from build123d import *

# Parameters (mm, degrees)
BOSS_EXTRUDE1_DEPTH = 20
SKETCH2_R           = 15.01
BOSS_EXTRUDE2_DEPTH = 20
CHAMFER1_SIZE       = 1
CHAMFER3_SIZE       = 1
SKETCH5_R           = 2.65
CUT_EXTRUDE2_DEPTH  = 40
FILLET3_R           = 5
SKETCH6_R           = 3.65
CUT_EXTRUDE3_DEPTH  = 8
CHAMFER4_SIZE       = 0.5
SKETCH10_R          = 15.01
BOSS_EXTRUDE5_DEPTH = 20
CHAMFER5_SIZE       = 1
SKETCH11_R          = 2.0099999999999967
CUT_EXTRUDE5_DEPTH  = 40
SKETCH12_R          = 2.0000000000000018
SKETCH12_R_2        = 2.000000000000005
SKETCH12_R_3        = 1.9999999999999967
CUT_EXTRUDE6_DEPTH  = 19.999999999999996


with BuildPart() as part:
    # Sketch1 → Boss-Extrude1 (new body)
    with BuildSketch(Plane(origin=(0, 0, 0), x_dir=(1, 0, 0), z_dir=(0, 1, 0))):
        with BuildLine():
            ThreePointArc((-23, 0), (1.41e-15, -22.999999999999982), (23, 0))
            ThreePointArc((23, 0), (17.845208734768505, 58.18386045047181), (20.033890701411753, 116.55459936267802))
            ThreePointArc((20.033890701411753, 116.55459936267802), (21.27316153822275, 124.05347023326534), (23.45051159720983, 131.33550314045155))
            ThreePointArc((23.45051159720983, 131.33550314045155), (-2.067e-14, 165.00000000000006), (-23.45051159720983, 131.3355031404515))
            ThreePointArc((-23.45051159720983, 131.3355031404515), (-21.27316153822273, 124.05347023326526), (-20.033890701411725, 116.55459936267786))
            ThreePointArc((-20.033890701411725, 116.55459936267786), (-17.845208734768505, 58.1838604504716), (-23, 0))
        make_face()
    extrude(amount=BOSS_EXTRUDE1_DEPTH)

    # Sketch2 → Boss-Extrude2 (add)
    with BuildSketch(Plane(origin=(0, 20, 0), x_dir=(1, 0, 0), z_dir=(0, 1, 0))):
        with Locations(Location((0, 0, 0), (0, 0, 90))):
            Circle(SKETCH2_R)
    extrude(amount=BOSS_EXTRUDE2_DEPTH)

    # Chamfer1
    chamfer1_edges = [part.edges().sort_by_distance(p)[0] for p in [
        (-2.76e-15, 40, 15.01),
    ]]
    chamfer(chamfer1_edges, length=CHAMFER1_SIZE)

    # Chamfer3
    # the kernel refuses this chamfer: 1 mm, written as the material it adds along each edge
    with BuildSketch(Plane(origin=(0, 20, 0), x_dir=(6e-17, 0, -1), z_dir=(1, 0, 6e-17))) as chamfer3_piece_1:
        Polygon((15.01, CHAMFER3_SIZE), (15.01 + CHAMFER3_SIZE, 0), (15.01, 0), align=None)
    revolve(axis=Axis((0, 20, 0), (0, 1, 0)))
    # the kernel refuses this chamfer: 1 mm, written as the material it takes off along each edge
    with BuildSketch(Plane(origin=(-79.73173943051358, 20, -110.54071067753486), x_dir=(0.9380204638883933, 0, -0.3465798743819428), z_dir=(-0.3465798743819428, 0, -0.9380204638883933))) as chamfer3_2_piece_1:
        Polygon((60.00000000000017 + CHAMFER3_SIZE, 0), (60.00000000000017, CHAMFER3_SIZE), (60.00000000000017, 0), align=None)
    revolve(axis=Axis((-79.73173943051358, 20, -110.54071067753486), (0, -1, 0)), revolution_arc=14.525766875036835, mode=Mode.SUBTRACT)
    with BuildSketch(Plane(origin=(-482.16572850262514, 20, -70.00000000000004), x_dir=(0.9949641454850282, 0, -0.1002314780857173), z_dir=(-0.1002314780857173, 0, -0.9949641454850282))) as chamfer3_2_piece_2:
        Polygon((464.4708454051196 + CHAMFER3_SIZE, 0), (464.4708454051196, CHAMFER3_SIZE), (464.4708454051196, 0), align=None)
    revolve(axis=Axis((-482.16572850262514, 20, -70.00000000000004), (0, -1, 0)), revolution_arc=14.737763084908373, mode=Mode.SUBTRACT)
    with BuildSketch(Plane(origin=(0, 20, -1.599e-14), x_dir=(-0.9937354343699007, 0, -0.11175816067592001), z_dir=(0.11175816067592001, 0, -0.9937354343699007))) as chamfer3_2_piece_3:
        Polygon((23.000000000000004 - CHAMFER3_SIZE, 0), (23.000000000000004, -CHAMFER3_SIZE), (23.000000000000004, 0), align=None)
    revolve(axis=Axis((0, 20, -1.599e-14), (0, 1, 0)), revolution_arc=192.83335153216495, mode=Mode.SUBTRACT)
    with BuildSketch(Plane(origin=(482.16572850261997, 20, -69.99999999999986), x_dir=(-0.9877285445231084, 0, 0.15618041597544133), z_dir=(0.15618041597544133, 0, 0.9877285445231084))) as chamfer3_2_piece_4:
        Polygon((464.4708454051149 + CHAMFER3_SIZE, 0), (464.47084540511446, CHAMFER3_SIZE), (464.4708454051149, 0), align=None)
    revolve(axis=Axis((482.16572850261997, 20, -69.99999999999986), (0, -1, 0)), revolution_arc=14.737763084908554, mode=Mode.SUBTRACT)
    with BuildSketch(Plane(origin=(79.7317394305139, 20, -110.54071067753493), x_dir=(-0.9949641454850281, 0, -0.10023147808571735), z_dir=(-0.10023147808571735, 0, 0.9949641454850281))) as chamfer3_2_piece_5:
        Polygon((60.000000000000455 + CHAMFER3_SIZE, 0), (60.000000000000455, CHAMFER3_SIZE), (60.000000000000455, 0), align=None)
    revolve(axis=Axis((79.7317394305139, 20, -110.54071067753493), (0, -1, 0)), revolution_arc=14.525766875036666, mode=Mode.SUBTRACT)
    with BuildSketch(Plane(origin=(9.77e-15, 20, -140.00000000000006), x_dir=(0.9380204638883942, 0, 0.3465798743819405), z_dir=(-0.3465798743819405, 0, 0.9380204638883942))) as chamfer3_2_piece_6:
        Polygon((24.999999999999982 - CHAMFER3_SIZE, 0), (24.999999999999982, -CHAMFER3_SIZE), (24.999999999999982, 0), align=None)
    revolve(axis=Axis((9.77e-15, 20, -140.00000000000006), (0, 1, 0)), revolution_arc=220.55653408148345, mode=Mode.SUBTRACT)

    # Sketch5 → Cut-Extrude2 (cut)
    with BuildSketch(Plane(origin=(0, 40, 0), x_dir=(1, 0, 0), z_dir=(0, 1, 0))):
        with Locations(Location((0, 0, 0), (0, 0, 270))):
            Circle(SKETCH5_R)
    extrude(amount=-CUT_EXTRUDE2_DEPTH, mode=Mode.SUBTRACT)

    # Fillet3
    # the kernel refuses this fillet: 5 mm, written as the material it takes off along each edge
    with BuildSketch(Plane(origin=(482.16572850261997, 0, -69.99999999999986), x_dir=(-0.9868985080370148, 0, 0.1613422909045059), z_dir=(0.1613422909045059, 0, 0.9868985080370148))) as fillet3_piece_1:
        with BuildLine():
            CenterArc((464.4708454051144 + FILLET3_R, -FILLET3_R), FILLET3_R, 89.99999999999935, 90.00000000000068)
            Line((464.4708454051144 + FILLET3_R, 8.9e-16), (464.4708454051144 + FILLET3_R, FILLET3_R * 0.02))
            Line((464.4708454051144 + FILLET3_R, FILLET3_R * 0.02), (464.4708454051144 - FILLET3_R * 0.02, FILLET3_R * 0.02))
            Line((464.4708454051144 - FILLET3_R * 0.02, FILLET3_R * 0.02), (464.4708454051144 - FILLET3_R * 0.02, -FILLET3_R))
            Line((464.4708454051144 - FILLET3_R * 0.02, -FILLET3_R), (464.4708454051144, -FILLET3_R))
        make_face()
    revolve(axis=Axis((482.16572850261997, 0, -69.99999999999986), (0, -1, 0)), revolution_arc=15.03731633345655, mode=Mode.SUBTRACT)
    with BuildSketch(Plane(origin=(0, 0, -1.599e-14), x_dir=(-0.9763879588864252, 0, -0.21602442857603077), z_dir=(0.21602442857603077, 0, -0.9763879588864252))) as fillet3_piece_2:
        with BuildLine():
            CenterArc((23 - FILLET3_R, FILLET3_R), FILLET3_R, 269.99999999999994, 90.00000000000006)
            Line((23 - FILLET3_R, -8.9e-16), (23 - FILLET3_R, -FILLET3_R * 0.02))
            Line((23 - FILLET3_R, -FILLET3_R * 0.02), (23 + FILLET3_R * 0.02, -FILLET3_R * 0.02))
            Line((23 + FILLET3_R * 0.02, -FILLET3_R * 0.02), (23 + FILLET3_R * 0.02, FILLET3_R))
            Line((23 + FILLET3_R * 0.02, FILLET3_R), (23.000000000000004, FILLET3_R))
        make_face()
    revolve(axis=Axis((0, 0, -1.599e-14), (0, 1, 0)), revolution_arc=204.95127041750123, mode=Mode.SUBTRACT)
    with BuildSketch(Plane(origin=(-482.16572850262514, 0, -70.00000000000004), x_dir=(0.9949641454850282, 0, -0.1002314780857173), z_dir=(-0.1002314780857173, 0, -0.9949641454850282))) as fillet3_piece_3:
        with BuildLine():
            CenterArc((464.4708454051196 + FILLET3_R, -FILLET3_R), FILLET3_R, 90, 90)
            Line((464.4708454051196 + FILLET3_R, 8.9e-16), (464.4708454051196 + FILLET3_R, FILLET3_R * 0.02))
            Line((464.4708454051196 + FILLET3_R, FILLET3_R * 0.02), (464.4708454051196 - FILLET3_R * 0.02, FILLET3_R * 0.02))
            Line((464.4708454051196 - FILLET3_R * 0.02, FILLET3_R * 0.02), (464.4708454051196 - FILLET3_R * 0.02, -FILLET3_R))
            Line((464.4708454051196 - FILLET3_R * 0.02, -FILLET3_R), (464.4708454051196, -FILLET3_R))
        make_face()
    revolve(axis=Axis((-482.16572850262514, 0, -70.00000000000004), (0, -1, 0)), revolution_arc=15.037316333456364, mode=Mode.SUBTRACT)
    with BuildSketch(Plane(origin=(-79.73173943051358, 0, -110.54071067753486), x_dir=(0.9380204638883933, 0, -0.3465798743819428), z_dir=(-0.3465798743819428, 0, -0.9380204638883933))) as fillet3_piece_4:
        with BuildLine():
            CenterArc((60.00000000000017 + FILLET3_R, -FILLET3_R), FILLET3_R, 90, 90)
            Line((60.00000000000017 + FILLET3_R, 8.9e-16), (60.00000000000017 + FILLET3_R, FILLET3_R * 0.02))
            Line((60.00000000000017 + FILLET3_R, FILLET3_R * 0.02), (60.00000000000017 - FILLET3_R * 0.02, FILLET3_R * 0.02))
            Line((60.00000000000017 - FILLET3_R * 0.02, FILLET3_R * 0.02), (60.00000000000017 - FILLET3_R * 0.02, -FILLET3_R))
            Line((60.00000000000017 - FILLET3_R * 0.02, -FILLET3_R), (60.00000000000018, -FILLET3_R))
        make_face()
    revolve(axis=Axis((-79.73173943051358, 0, -110.54071067753486), (0, -1, 0)), revolution_arc=14.525766875036835, mode=Mode.SUBTRACT)
    with BuildSketch(Plane(origin=(9.77e-15, 0, -140.00000000000006), x_dir=(0.9380204638883942, 0, 0.3465798743819405), z_dir=(-0.3465798743819405, 0, 0.9380204638883942))) as fillet3_piece_5:
        with BuildLine():
            CenterArc((24.999999999999982 - FILLET3_R, FILLET3_R), FILLET3_R, 270, 90)
            Line((24.999999999999982 - FILLET3_R, -8.9e-16), (24.999999999999982 - FILLET3_R, -FILLET3_R * 0.02))
            Line((24.999999999999982 - FILLET3_R, -FILLET3_R * 0.02), (24.999999999999982 + FILLET3_R * 0.02, -FILLET3_R * 0.02))
            Line((24.999999999999982 + FILLET3_R * 0.02, -FILLET3_R * 0.02), (24.999999999999982 + FILLET3_R * 0.02, FILLET3_R))
            Line((24.999999999999982 + FILLET3_R * 0.02, FILLET3_R), (24.999999999999986, FILLET3_R))
        make_face()
    revolve(axis=Axis((9.77e-15, 0, -140.00000000000006), (0, 1, 0)), revolution_arc=220.55653408148345, mode=Mode.SUBTRACT)
    with BuildSketch(Plane(origin=(79.7317394305139, 0, -110.54071067753493), x_dir=(-0.9949641454850281, 0, -0.10023147808571735), z_dir=(-0.10023147808571735, 0, 0.9949641454850281))) as fillet3_piece_6:
        with BuildLine():
            CenterArc((60.000000000000455 + FILLET3_R, -FILLET3_R), FILLET3_R, 90, 90)
            Line((60.000000000000455 + FILLET3_R, 8.9e-16), (60.000000000000455 + FILLET3_R, FILLET3_R * 0.02))
            Line((60.000000000000455 + FILLET3_R, FILLET3_R * 0.02), (60.000000000000455 - FILLET3_R * 0.02, FILLET3_R * 0.02))
            Line((60.000000000000455 - FILLET3_R * 0.02, FILLET3_R * 0.02), (60.000000000000455 - FILLET3_R * 0.02, -FILLET3_R))
            Line((60.000000000000455 - FILLET3_R * 0.02, -FILLET3_R), (60.000000000000455, -FILLET3_R))
        make_face()
    revolve(axis=Axis((79.7317394305139, 0, -110.54071067753493), (0, -1, 0)), revolution_arc=14.525766875036666, mode=Mode.SUBTRACT)

    # Sketch6 → Cut-Extrude3 (cut)
    with BuildSketch(Plane.XZ):
        with Locations(Location((0, 0, 0), (0, 0, 270))):
            Circle(SKETCH6_R)
    extrude(amount=-CUT_EXTRUDE3_DEPTH, mode=Mode.SUBTRACT)

    # Chamfer4
    chamfer4_edges = [part.edges().sort_by_distance(p)[0] for p in [
        (1.12e-15, 0, 3.65),
    ]]
    chamfer(chamfer4_edges, length=CHAMFER4_SIZE)

    # Sketch10 → Boss-Extrude5 (add)
    with BuildSketch(Plane(origin=(0, 20, 0), x_dir=(1, 0, 0), z_dir=(0, 1, 0))):
        with Locations(Location((0, 140.00000000000009, 0), (0, 0, 90))):
            Circle(SKETCH10_R)
    extrude(amount=BOSS_EXTRUDE5_DEPTH)

    # Chamfer5
    chamfer5_edges = [part.edges().sort_by_distance(p)[0] for p in [
        (-2.76e-15, 20, -124.99000000000008),
        (-2.76e-15, 40, -124.99000000000008),
    ]]
    chamfer(chamfer5_edges, length=CHAMFER5_SIZE)

    # Sketch11 → Cut-Extrude5 (cut)
    with BuildSketch(Plane(origin=(0, 40, 0), x_dir=(1, 0, 0), z_dir=(0, 1, 0))):
        with Locations(Location((0, 140.00000000000009, 0), (0, 0, 270))):
            Circle(SKETCH11_R)
    extrude(amount=-CUT_EXTRUDE5_DEPTH, mode=Mode.SUBTRACT)

    # Sketch12 → Cut-Extrude6 (cut)
    with BuildSketch(Plane(origin=(0, 40, 0), x_dir=(1, 0, 0), z_dir=(0, 1, 0))):
        with Locations(Location((-6.500000000000021, 146.50000000000014, 0), (0, 0, 270))):
            Circle(SKETCH12_R)
        with Locations(Location((-6.4999999999999885, 133.5000000000001, 0), (0, 0, 270))):
            Circle(SKETCH12_R)
        with Locations(Location((6.500000000000011, 133.50000000000009, 0), (0, 0, 90))):
            Circle(SKETCH12_R_2)
        with Locations(Location((6.499999999999978, 146.5000000000001, 0), (0, 0, 90))):
            Circle(SKETCH12_R_3)
    extrude(amount=-CUT_EXTRUDE6_DEPTH, mode=Mode.SUBTRACT)


solid = part.part
Verification items for the finished model (mm, model axes). A direction names the side the tool comes from. Coordinates: 2 decimals unless noted, no trailing zeros. Loops run counter-clockwise (first coordinate to the right, second up) from the corner with the lowest first, then second, coordinate; pieces in that order, holes last. Notation, with made-up numbers: M 52,20.25 L 109,20.25 A10 ccw 109,30.25 Z; hole C 57.5,25.25 d10. An arc over 180 degrees is marked long. One line per item, written item: value.
1. Section check A-A on y = 16.5. Record the cut outline in (x, z).
Answers follow:
outline: M -23.45,-131.34 A25 ccw long 23.45,-131.34 A60 cw 20.03,-116.55 A464.47 cw 23,0 A23 ccw -23,0 A464.47 cw -20.03,-116.55 A60 cw Z; hole C 0,0 d5.3; hole C 0,-140 d4.02
2. Mould release check, pull along Z, two halves, no side actions. Record for faces 1 (the flat face through (6, 20, -133)), 2 (the cylindrical face through (-0.506, 11.902, 22.994)), 3 (the flat face through (0, 20, -72)), 4 (the flat face through (0, 40, -143)): pulls with the +Z half, pulls with the -Z half, needs draft (parallel to the pull), parting line crosses it, or undercut.
Answers follow:
face 1: undercut
face 2: pulls with the +Z half
face 3: undercut
face 4: needs draft
3. Material ranges on line 1 along X through (y, z) = (31.5, 0); line 2 along Z through (x, y) = (7, 33.5); line 3 along X through (y, z) = (24.75, -133.5), recorded low to high. Write a range as from..to.
Answers follow:
line 1: -15.01..-2.65, 2.65..15.01
line 2: -153.28..-148.44, -144.56..-135.44, -131.56..-126.72, -13.28..13.28
line 3: -13.53..-8.5, -4.5..4.5, 8.5..13.53
4. Section check B-B on x = 0. Give the number of separate pieces and of enclosed holes in the cut face, plus the area to 3 significant figures.
Answers follow:
separate pieces: 3
enclosed holes: 0
area: 4,560 mm^2
5. Set-up check for faces 5 (the cylindrical face through (-6.412, 30.14, -135.498)), 6 (the cylindrical face through (-1.4, 4.2, -3.37)), 7 (the cylindrical face through (-21.297, 11.902, -124.157)): record each of +Z, -Z, +X, -X, +Y, -Y from which the full face is reachable in a straight line by a thin tool's end or side.
Answers follow:
face 5: +Y
face 6: -Y
face 7: -X, +Y, -Y
6. Gauge pin test, flat ends, axial feed: P1, Ø7, axis at x = 0, z = 0, coming from the -Y side; P2, Ø1, axis at x = -5.5, z = -17.5, coming from the +Y side; P3, Ø4, axis at x = 11, y = 9.5, coming from the +Z side. Record the tip position at first contact, or that the pin passes through.
Answers follow:
P1: y = 8
P2: y = 20
P3: z = 21.17
